from build123d import *

# Parameters (mm, degrees)
F1_DEPTH = 121
F3_DEPTH = 2


with BuildPart() as f1:
    # F0 (on Front) → F1 (new body)
    with BuildSketch(Plane.XZ):
        with BuildLine():
            Line((77.5, 75), (-77.5, 75))
            ThreePointArc((-77.5, 75), (-81.035534, 73.535534), (-82.5, 70))
            Line((-82.5, 70), (-82.5, -70))
            ThreePointArc((-82.5, -70), (-81.035534, -73.535534), (-77.5, -75))
            Line((-77.5, -75), (77.5, -75))
            ThreePointArc((77.5, -75), (81.035534, -73.535534), (82.5, -70))
            Line((82.5, -70), (82.5, 70))
            ThreePointArc((82.5, 70), (81.035534, 73.535534), (77.5, 75))
        make_face()
        with BuildLine():
            ThreePointArc((-72.5, 60), (-71.035534, 63.535534), (-67.5, 65))
            Line((-67.5, 65), (67.5, 65))
            ThreePointArc((67.5, 65), (71.035534, 63.535534), (72.5, 60))
            Line((72.5, 60), (72.5, -60))
            ThreePointArc((72.5, -60), (71.035534, -63.535534), (67.5, -65))
            Line((67.5, -65), (-67.5, -65))
            ThreePointArc((-67.5, -65), (-71.035534, -63.535534), (-72.5, -60))
            Line((-72.5, -60), (-72.5, 60))
        make_face(mode=Mode.SUBTRACT)
    extrude(amount=F1_DEPTH)

    # F2 (on Front) → F3 (join)
    with BuildSketch(Plane.XZ):
        with BuildLine():
            Line((77.622953, 74.877053), (-77.622953, 74.877053))
            ThreePointArc((-77.622953, 74.877053), (-81.158487, 73.412587), (-82.622953, 69.877053))
            Line((-82.622953, 69.877053), (-82.622953, -69.877053))
            ThreePointArc((-82.622953, -69.877053), (-81.158487, -73.412587), (-77.622953, -74.877053))
            Line((-77.622953, -74.877053), (77.622953, -74.877053))
            ThreePointArc((77.622953, -74.877053), (81.158487, -73.412587), (82.622953, -69.877053))
            Line((82.622953, -69.877053), (82.622953, 69.877053))
            ThreePointArc((82.622953, 69.877053), (81.158487, 73.412587), (77.622953, 74.877053))
        make_face()
    extrude(amount=F3_DEPTH)


solid = f1.part
Can you work these out from the model? Positions are in its coordinate system, mm. Give positions to 0.01 mm unless a question says otherwise; leave off trailing zeros. Order: outer loops, then holes, each group sorted by start corner. A loop starts at its lowest first (then second) coordinate and runs counter-clockwise, first axis right, second up. Notation, with made-up numbers: M 67,81.5 L 124,81.5 A24 ccw 124,92.5 Z; hole C 79,67.5 d2. An arc over 180 degrees is marked long. One line per question, with ' | ' between items.
Item 1: Please list where these lines run through material, in increasing order: L1, parallel to X at y = -26, z = 48; L2, parallel to Z at x = 51, y = -12; L3, parallel to Y at x = 41.5, z = -30.5.
Answer block:
L1: x = -82.5 to -72.5, 72.5 to 82.5 | L2: z = -75 to -65, 65 to 75 | L3: y = -2 to 0
Item 2: Suppose I cut it at A-A, the plane y = -95.5. Write out the boundary of the cut face in (x, z), then the cut area to 3 significant figures.
Answer block:
outline: M -82.5,-70 A5 ccw -77.5,-75 L 77.5,-75 A5 ccw 82.5,-70 L 82.5,70 A5 ccw 77.5,75 L -77.5,75 A5 ccw -82.5,70 Z; hole M -72.5,-60 A5 ccw -67.5,-65 L 67.5,-65 A5 ccw 72.5,-60 L 72.5,60 A5 ccw 67.5,65 L -67.5,65 A5 ccw -72.5,60 Z | area: 5,900 mm2
Item 3: We'd pull the mould along X, two halves only. Please class faces 1 (the face through (-82.5, -61, 1)), 2 (the face through (0, -121, 67)), 3 (the face through (1, -61, -65)): released by +X, released by -X, zero draft, split by the parting line, or undercut.
Answer block:
face 1: released by -X | face 2: zero draft | face 3: undercut
Item 4: I'm going to push flat-ended pins straight in: pin 1 Ø4 at (y, z) = (-80, -22.5) entering from +X; pin 2 Ø4 at (x, z) = (-29.5, -40.5) entering from -Y; pin 3 Ø1.5 at (y, z) = (-49.5, -25) entering from -X. Where does each tip first touch, or does it pass through?
Answer block:
pin 1: stops at x = 82.5 | pin 2: stops at y = -2 | pin 3: stops at x = -82.5
Item 5: Suppose I cut it at B-B, the plane z = -32.5. Write out the boundary of the cut face in (x, y).
Answer block:
outline: M -82.62,-2 L -82.5,-2 L -82.5,-121 L -72.5,-121 L -72.5,-2 L 72.5,-2 L 72.5,-121 L 82.5,-121 L 82.5,-2 L 82.62,-2 L 82.62,0 L -82.62,0 Z
Item 6: Suppose I cut it at C-C, the plane x = 36. Write out the boundary of the cut face in (y, z).
Answer block:
outline: M -121,-75 L 0,-75 L 0,75 L -121,75 L -121,65 L -2,65 L -2,-65 L -121,-65 Z
